CAD build for the part. Positions are in the model's coordinates, mm. A direction names the side the tool comes from. Give positions to 0.01 mm unless a question says otherwise; leave off trailing zeros. Write each loop counter-clockwise with the first axis right and the second up, starting at its lowest first coordinate (ties: lowest second). Pieces come first, ordered by that corner, then holes. Notation, with made-up numbers: M -40,1 L -28,1 A29 cw -28,24 Z; hole C -7.75,65.25 d10. An arc over 180 degrees is marked long. One line per question, with ' | ' between items. Start each with the question number.
1. Flat gauge pins, fed straight in: pin 1 (0.8 mm diameter, centred on y = 6, z = -13, fed in from +X); pin 2 (1 mm diameter, centred on x = -21, y = 16, fed in from +Z); pin 3 (1.7 mm diameter, centred on y = 6.5, z = -13.5, fed in from -X). Where does each tip first touch, or does it go through?
2. Cut at A-A, the plane y = 8.75. Write the cut outline in (x, z), then the cut area to 3 significant figures.
3. Cut at C-C, the plane y = 10.75. Write the cut outline in (x, z), then the cut area to 3 significant figures.
4. Cut at B-B, the plane y = 13.75. Write the cut outline in (x, z).
5. Which spindle directions (+Z, -Z, +X, -X, +Y, -Y) get a long thin tool onto all of the face, cutting with end or side? Do faces 4 (the face through (-20, 5, -12.228)), 5 (the face through (-17, 5, -10.728)), 6 (the face through (-20.765, 4.684, -11.488)), 7 (the face through (-17, 5, -12.228)), 8 (the face through (-16.947, 15.302, -10.941)). Say none if no direction does.
6. Pull direction X, two halves, no side cores. Call faces 1 (the face through (-20.24, 15.3, -12.12)), 2 (the face through (-15.662, 14.444, -14.377)), 3 (the face through (-19.115, 5, -13)): released by +X, released by -X, zero draft, split by the parting line, or undercut.
7. Wall check: L1, parallel to Y at x = -20.5, z = -9.5; L2, parallel to X at y = 1.5, z = -13.5; L3, parallel to Z at x = -19.5, y = 14.25. Give the ranges that are in metal, low to high.
```python
from build123d import *

# Parameters (mm, degrees)
RESSALTO_EXTRUS_O1_DEPTH = 10
ESBO_O7_R                = 4
RESSALTO_EXTRUS_O3_DEPTH = 9
CORTE_EXTRUS_O2_DEPTH    = 7.5
FILETE9_R                = 0.5


with BuildPart() as part:
    # Esboço1 → Ressalto-extrusão1 (new body)
    with BuildSketch(Plane(origin=(0, 0, 0), x_dir=(1, 0, 0), z_dir=(0, 1, 0))):
        with BuildLine():
            Line((-16.085684063, 12.227593462), (-17.615486686, 12.227593462))
            Line((-17.615486686, 12.227593462), (-17.615486686, 13.727593462))
            Line((-17.615486686, 13.727593462), (-17.615486686, 13.757396085))
            ThreePointArc((-17.615486686, 13.757396085), (-18.365486686, 13.877593462), (-19.115486686, 13.757396085))
            Line((-19.115486686, 13.757396085), (-19.115486686, 13.727593462))
            Line((-19.115486686, 13.727593462), (-19.115486686, 12.227593462))
            Line((-19.115486686, 12.227593462), (-20.615486686, 12.227593462))
            Line((-20.615486686, 12.227593462), (-20.645289309, 12.227593462))
            ThreePointArc((-20.645289309, 12.227593462), (-20.765486686, 11.477593462), (-20.645289309, 10.727593462))
            Line((-20.645289309, 10.727593462), (-20.615486686, 10.727593462))
            Line((-20.615486686, 10.727593462), (-19.115486686, 10.727593462))
            Line((-19.115486686, 10.727593462), (-19.115486686, 9.227593462))
            Line((-19.115486686, 9.227593462), (-19.115486686, 9.197790839))
            ThreePointArc((-19.115486686, 9.197790839), (-18.365486686, 9.077593462), (-17.615486686, 9.197790839))
            Line((-17.615486686, 9.197790839), (-17.615486686, 9.227593462))
            Line((-17.615486686, 9.227593462), (-17.615486686, 10.727593462))
            Line((-17.615486686, 10.727593462), (-16.085684063, 10.727593462))
            ThreePointArc((-16.085684063, 10.727593462), (-15.965486686, 11.477593462), (-16.085684063, 12.227593462))
        make_face()
    extrude(amount=RESSALTO_EXTRUS_O1_DEPTH)

    # Esboço7 → Ressalto-extrusão3 (add)
    with BuildSketch(Plane(origin=(0, 10, 0), x_dir=(1, 0, 0), z_dir=(0, 1, 0))):
        with Locations(Location((-18.365486686, 11.428442315, 0), (0, 0, 270))):
            Circle(ESBO_O7_R)
    extrude(amount=RESSALTO_EXTRUS_O3_DEPTH)

    # Esboço9 → Corte-extrusão2 (cut)
    with BuildSketch(Plane(origin=(0, 19, 0), x_dir=(1, 0, 0), z_dir=(0, 1, 0))):
        with BuildLine():
            Line((-17.35582754, 9.702004246), (-16.526382122, 12.214377685))
            ThreePointArc((-16.526382122, 12.214377685), (-20.264662492, 12.055444115), (-17.35582754, 9.702004246))
        make_face()
    extrude(amount=-CORTE_EXTRUS_O2_DEPTH, mode=Mode.SUBTRACT)

    # Filete9
    filete9_edges = [part.edges().sort_by_distance(p)[0] for p in [
        (-20.765486686, 10, -11.477593462),
        (-19.880387997, 10, -10.727593462),
        (-19.115486686, 10, -9.96269215),
        (-18.365486686, 10, -9.077593462),
        (-17.615486686, 10, -9.96269215),
        (-16.850585374, 10, -10.727593462),
        (-15.965486686, 10, -11.477593462),
        (-18.365486686, 10, -15.428442315),
        (-18.365486686, 19, -15.428442315),
        (-16.850585374, 10, -12.227593462),
        (-17.615486686, 10, -12.992494773),
        (-19.880387997, 10, -12.227593462),
        (-18.365486686, 10, -13.877593462),
        (-19.115486686, 10, -12.992494773),
    ]]
    fillet(filete9_edges, radius=FILETE9_R)


solid = part.part
```
Here are the results:
1) pin 1: x = -17.62 | pin 2: z = -8.05 | pin 3: x = -19.12
2) outline: M -20.65,-12.23 L -19.12,-12.23 L -19.12,-13.76 A2.4 ccw -17.62,-13.76 L -17.62,-12.23 L -16.09,-12.23 A2.4 ccw -16.09,-10.73 L -17.62,-10.73 L -17.62,-9.2 A2.4 ccw -19.12,-9.2 L -19.12,-10.73 L -20.65,-10.73 A2.4 ccw Z | area: 11.9 mm^2
3) outline: C -18.37,-11.43 d8 | area: 50.3 mm^2
4) outline: C -18.37,-11.43 d8; hole M -17.36,-9.7 A2 ccw long -16.53,-12.21 Z
5) face 4: -Z, -X, -Y | face 5: +Z, +X, -Y | face 6: -X, -Y | face 7: -Z, +X, -Y | face 8: +Y
6) face 1: undercut | face 2: split by the parting line | face 3: released by -X
7) L1: 10 to 19 | L2: -19.12 to -17.62 | L3: -15.26 to -13.08, -9.78 to -7.59
